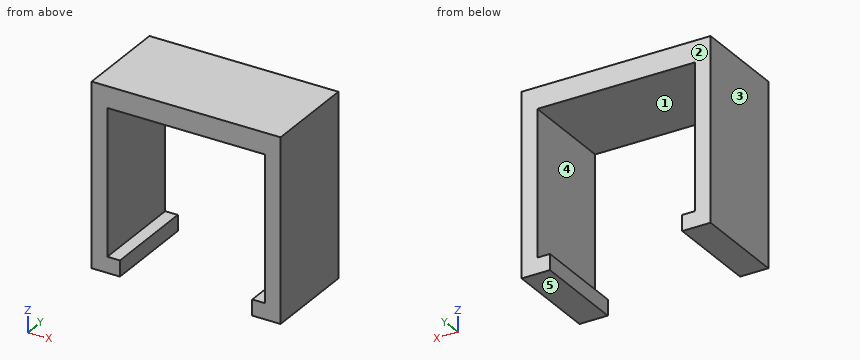
from build123d import *

# Parameters (mm, degrees)
F0_W      = 35
F0_H      = 15
F1_DEPTH  = 7.366
F2_W      = 5
F2_H      = 15
F3_DEPTH  = 28
F4_W      = 5
F4_H      = 15
F5_DEPTH  = 28
F7_W      = 15
F7_H      = 5
F8_DEPTH  = 2
F6_W      = 15
F6_H      = 5
F9_DEPTH  = 2
F10_DEPTH = 4
F11_DEPTH = 2.5
F12_DEPTH = 2.5
F13_DEPTH = 2.5


with BuildPart() as f1:
    # F0 (on Top) → F1 (new body)
    with BuildSketch(Plane.XY):
        with Locations((-18.1619706172, -22.7490997307)):
            Rectangle(F0_W, F0_H)
    extrude(amount=-F1_DEPTH)

    # F2 (on face) → F3 (join)
    with BuildSketch(Plane(origin=(0, 0, -7.366), x_dir=(1, 0, 0), z_dir=(0, 0, -1))):
        with Locations((-33.1619706172, 22.7490997307)):
            Rectangle(F2_W, F2_H)
    extrude(amount=F3_DEPTH)

    # F4 (on face) → F5 (join)
    with BuildSketch(Plane(origin=(0, 0, -7.366), x_dir=(1, 0, 0), z_dir=(0, 0, -1))):
        with Locations((-3.1619706172, 22.7490997307)):
            Rectangle(F4_W, F4_H)
    extrude(amount=F5_DEPTH)

    # F7 (on face) → F8 (join)
    with BuildSketch(Plane.YZ.offset(-30.6619706172)):
        with Locations((-22.7490997307, -32.866)):
            Rectangle(F7_W, F7_H)
    extrude(amount=F8_DEPTH)

    # F6 (on face) → F9 (join)
    with BuildSketch(Plane(origin=(-5.6619706172, 0, 0), x_dir=(0, -1, 0), z_dir=(-1, 0, 0))):
        with Locations((22.7490997307, -32.866)):
            Rectangle(F6_W, F6_H)
    extrude(amount=F9_DEPTH)

    # F10 (cut): a face of the model
    f10_faces = [f1.faces().sort_by_distance(p)[0] for p in [
        (-18.1619706172, -22.7490997307, 0),
    ]]
    extrude(f10_faces, amount=-F10_DEPTH, mode=Mode.SUBTRACT)

    # F11 (cut): a face of the model
    f11_faces = [f1.faces().sort_by_distance(p)[0] for p in [
        (-0.6619706172, -22.7490997307, -19.683),
    ]]
    extrude(f11_faces, amount=-F11_DEPTH, mode=Mode.SUBTRACT)

    # F12 (cut): a face of the model
    f12_faces = [f1.faces().sort_by_distance(p)[0] for p in [
        (-35.6619706172, -22.7490997307, -19.683),
    ]]
    extrude(f12_faces, amount=-F12_DEPTH, mode=Mode.SUBTRACT)

    # F13 (cut): faces of the model
    f13_faces = [f1.faces().sort_by_distance(p)[0] for p in [
        (-30.9119706172, -22.7490997307, -35.366),
        (-5.4119706172, -22.7490997307, -35.366),
    ]]
    extrude(f13_faces, amount=-F13_DEPTH, mode=Mode.SUBTRACT)


solid = f1.part
For this review, take the finished solid that the model builds, in its own axes (mm). Face numbers are marked on the shaded views. A direction names the side the tool comes from. Round coordinates to 2 decimals unless told otherwise and drop trailing zeros. Loops run counter-clockwise (first coordinate to the right, second up) from the corner with the lowest first, then second, coordinate; pieces in that order, holes last. Notation, with made-up numbers: (-34, 51.5) - (23, 51.5) arc R32 ccw to (23, 80.5) - close; hole circle Ø2 at (17.25, 87.25). An arc over 180 degrees is marked (long way). Put each result on its own line as item: value. Start each with the question number.
1. Mouldability with a two-part tool opening along X and no side actions: class the marked faces 1, 2 and 3 as +X half, -X half, draft (parallel to the pull), parting line (faces both ways), or undercut.
2. Consider section D-D on x = -24.5. State the section outline as (y, z) points, plus the area to 3 significant figures.
3. Consider section B-B on z = -14.5. State the section outline as (x, y) points, plus the area to 3 significant figures.
4. Consider section C-C on y = -27. State the section outline as (x, z) points, plus the area to 3 significant figures.
5. For the marked faces 4 and 5, list the 3-axis set-ups (+Z, -Z, +X, -X, +Y, -Y) from which the entire face can be reached by the end or side of a thin tool; tool diameter is ignored.
6. For probe 1 along X at (y, z) = (-21.25, -22); probe 2 along Z at (x, y) = (-7.5, -16.5); probe 3 along Z at (x, y) = (-25.75, -19.25), list the stretches that pass through material, from the lowest coordinate up. Write a range as [from, to].
7. Consider section A-A on x = -30. State the section outline as (y, z) points, plus the area to 3 significant figures.
Result sheet:
1. face 1: undercut
1. face 2: draft
1. face 3: -X half
2. outline: (-30.25, -7.37) - (-15.25, -7.37) - (-15.25, -4) - (-30.25, -4) - close
2. area: 50.5 mm^2
3. outline: (-33.16, -30.25) - (-30.66, -30.25) - (-30.66, -15.25) - (-33.16, -15.25) - close; (-5.66, -30.25) - (-3.16, -30.25) - (-3.16, -15.25) - (-5.66, -15.25) - close
3. area: 75.0 mm^2
4. outline: (-33.16, -32.87) - (-28.66, -32.87) - (-28.66, -30.37) - (-30.66, -30.37) - (-30.66, -7.37) - (-5.66, -7.37) - (-5.66, -30.37) - (-7.66, -30.37) - (-7.66, -32.87) - (-3.16, -32.87) - (-3.16, -4) - (-33.16, -4) - close
4. area: 238 mm^2
5. face 4: +Y, -Y
5. face 5: -Z, +X, -X, +Y, -Y
6. probe 1: [-33.16, -30.66], [-5.66, -3.16]
6. probe 2: [-32.87, -30.37], [-7.37, -4]
6. probe 3: [-7.37, -4]
7. outline: (-30.25, -32.87) - (-15.25, -32.87) - (-15.25, -30.37) - (-30.25, -30.37) - close; (-30.25, -7.37) - (-15.25, -7.37) - (-15.25, -4) - (-30.25, -4) - close
7. area: 88.0 mm^2
